from build123d import *

# Parameters (mm, degrees)
SKETCH1_R           = 32.5
BOSS_EXTRUDE1_DEPTH = 2
SKETCH2_R           = 32.5
BOSS_EXTRUDE2_DEPTH = 13
SKETCH6_W           = 71.390071862
SKETCH6_H           = 35.774890597
CUT_EXTRUDE4_DEPTH  = 13


with BuildPart() as part:
    # Sketch1 → Boss-Extrude1 (new body)
    with BuildSketch(Plane(origin=(0, 0, 0), x_dir=(1, 0, 0), z_dir=(0, 1, 0))):
        with Locations(Location((0, 0, 0), (0, 0, 270))):
            Circle(SKETCH1_R)
    extrude(amount=BOSS_EXTRUDE1_DEPTH)

    # Sketch2 → Boss-Extrude2 (add)
    with BuildSketch(Plane(origin=(0, 2, 0), x_dir=(1, 0, 0), z_dir=(0, 1, 0))):
        with Locations(Location((0, 0, 0), (0, 0, 270))):
            Circle(SKETCH2_R)
        with BuildLine():
            Line((2.6, -27.125679715), (2.6, -30))
            Line((2.6, -30), (-2.6, -30))
            Line((-2.6, -30), (-2.6, -27.125679715))
            ThreePointArc((-2.6, -27.125679715), (-19.268659787, -19.268659787), (-27.125679715, -2.6))
            Line((-27.125679715, -2.6), (-30, -2.6))
            Line((-30, -2.6), (-30, 2.6))
            Line((-30, 2.6), (-27.125679715, 2.6))
            ThreePointArc((-27.125679715, 2.6), (-19.268659787, 19.268659787), (-2.6, 27.125679715))
            Line((-2.6, 27.125679715), (-2.6, 30))
            Line((-2.6, 30), (2.6, 30))
            Line((2.6, 30), (2.6, 27.125679715))
            ThreePointArc((2.6, 27.125679715), (19.268659787, 19.268659787), (27.125679715, 2.6))
            Line((27.125679715, 2.6), (30, 2.6))
            Line((30, 2.6), (30, -2.6))
            Line((30, -2.6), (27.125679715, -2.6))
            ThreePointArc((27.125679715, -2.6), (19.268659787, -19.268659787), (2.6, -27.125679715))
        make_face(mode=Mode.SUBTRACT)
    extrude(amount=BOSS_EXTRUDE2_DEPTH)

    # Sketch6 → Cut-Extrude4 (cut)
    with BuildSketch(Plane(origin=(0, 15, 0), x_dir=(1, 0, 0), z_dir=(0, 1, 0))):
        with Locations((0.159709333, -17.887445299)):
            Rectangle(SKETCH6_W, SKETCH6_H)
    extrude(amount=-CUT_EXTRUDE4_DEPTH, mode=Mode.SUBTRACT)


solid = part.part
Here's how the part is built. I have some questions about the finished solid (model axes, mm). A direction names the side the tool comes from. Round coordinates to 2 decimals unless told otherwise and drop trailing zeros. Order: outer loops, then holes, each group sorted by start corner. A loop starts at its lowest first (then second) coordinate and runs counter-clockwise, first axis right, second up. Notation, with made-up numbers: (20.25, 7.5) -> (50.25, 7.5) arc R13 ccw to (50.25, 18.5) -> close; hole circle Ø10 at (-29.75, 83.25). An arc over 180 degrees is marked (long way). Use CSV: the item, a comma, the result in double quotes.
1. I want a section at B-B on x = 0. List the corners of the cut face in (y, z) for me, and give its area (4 significant figures).
Recorded:
outline,"(0, -32.5) -> (15, -32.5) -> (15, -30) -> (2, -30) -> (2, 32.5) -> (0, 32.5) -> close"
area,"162.5 mm2"
2. I want a section at C-C on z = -10. List the corners of the cut face in (x, y) for me, and give its area (3 significant figures).
Recorded:
outline,"(-30.92, 0) -> (30.92, 0) -> (30.92, 15) -> (25.35, 15) -> (25.35, 2) -> (-25.35, 2) -> (-25.35, 15) -> (-30.92, 15) -> close"
area,"269 mm2"
3. I want a section at A-A on y = 6.25. List the corners of the cut face in (x, z) for me, and give its area (3 significant figures).
Recorded:
outline,"(-32.5, 0) arc R32.5 ccw to (32.5, 0) -> (30, 0) -> (30, -2.6) -> (27.13, -2.6) arc R27.25 cw to (2.6, -27.13) -> (2.6, -30) -> (-2.6, -30) -> (-2.6, -27.13) arc R27.25 cw to (-27.13, -2.6) -> (-30, -2.6) -> (-30, 0) -> close"
area,"464 mm2"
4. Thinking about a two-plate mould opening in X: for faces 1 (the face through (1.43, 7.4, -32.47)), 2 (the face through (0, 0, 0)), 3 (the face through (19.082, 8.409, -19.454)), 4 (the face through (2.6, 8, -29)), which applies, pulls with the +X half, pulls with the -X half, needs draft (parallel to the pull), parting line crosses it, or undercut?
Recorded:
face 1,"parting line crosses it"
face 2,"needs draft"
face 3,"undercut"
face 4,"undercut"
5. Which directions (+Z, -Z, +X, -X, +Y, -Y) give clear straight access to the entire face, cutting with the end or side of a thin tool? Please do faces 5 (the face through (31, 9, 0)), 6 (the face through (-19.454, 8.409, -19.082)), 7 (the face through (7, 15, -27)).
Recorded:
face 5,"+Z, +X, -X, +Y"
face 6,"+Z, +Y"
face 7,"+Z, -Z, +X, -X, +Y"
6. I want a section at D-D on x = 16. List the corners of the cut face in (y, z) for me.
Recorded:
outline,"(0, -28.29) -> (15, -28.29) -> (15, -22.06) -> (2, -22.06) -> (2, 28.29) -> (0, 28.29) -> close"
7. I'm going to push flat-ended pins straight in: P1, Ø2, axis at x = -5, y = 10.5, coming from the +Z side; P2, Ø1.5, axis at y = 5.5, z = -16.5, coming from the -X side; P3, Ø1.5, axis at x = -1, y = 9, coming from the -Z side. Where does each tip first touch, or does it pass through?
Recorded:
P1,"stops at z = -26.58"
P2,"stops at x = -28.43"
P3,"stops at z = -32.5"
8. I need wall thicknesses on line 1 along Y through (x, z) = (-27, -2); line 2 along X through (y, z) = (2.5, -29.5); line 3 along X through (y, z) = (14, -3). Which ranges of each line are inside material? Lowest first, please.
Recorded:
line 1,"y = 0 to 2"
line 2,"x = -13.64 to -2.6, 2.6 to 13.64"
line 3,"x = -32.36 to -27.08, 27.08 to 32.36"
